from build123d import *

# Parameters (mm, degrees)
SKETCH1_W               = 339.725
SKETCH1_H               = 88.9
BOSS_EXTRUDE1_DEPTH     = 6.35
F_1_4_CLEARANCE_HOLE1_D = 6.7564
FILLET1_R               = 3.175


with BuildPart() as part:
    # Sketch1 → Boss-Extrude1 (new body)
    with BuildSketch(Plane(origin=(0, 0, 0), x_dir=(-1, 0, 0), z_dir=(0, 0, -1))):
        Rectangle(SKETCH1_W, SKETCH1_H)
    extrude(amount=-BOSS_EXTRUDE1_DEPTH)

    # 1/4 Clearance Hole1 (through all)
    with Locations(Plane.XY.offset(6.35)):
        with Locations((-160.3375, 34.925), (-160.3375, -34.925), (160.3375, 34.925), (160.3375, -34.925)):
            Hole(F_1_4_CLEARANCE_HOLE1_D / 2)

    # Fillet1
    fillet1_edges = [part.edges().sort_by_distance(p)[0] for p in [
        (169.8625, 44.45, 3.175),
        (-169.8625, 44.45, 3.175),
        (-169.8625, -44.45, 3.175),
        (169.8625, -44.45, 3.175),
    ]]
    fillet(fillet1_edges, radius=FILLET1_R)


solid = part.part
Could you check a few things on this model? Use its own coordinates, in mm. Coordinates: 2 decimals unless noted, no trailing zeros. Answer in a Markdown table with one row per item. Add a question column.
(1) I need wall thicknesses on L1, parallel to X at y = 32, z = 4.25; L2, parallel to X at y = -37, z = 4.75. Which ranges of each line are inside material? Lowest first, please.
(2) Will this pin go through, and if not, where does the flat tip stop? pin 1 (5.5 mm diameter, centred on x = 160.34, y = 34.92, fed in from -Z).
(3) If we mould it in two halves opening along X, with no side actions, what happens to faces 1 (the face through (2, 1, 0)), 2 (the face through (-169.862, -1, 3)), 3 (the face through (-163.56, -33.91, 3.13))? For each: released by +X, released by -X, zero draft, split by the parting line, or undercut.
Results are:
| question | item | result |
|---|---|---|
| 1 | L1 | x = -169.86 to -162.03, -158.65 to 158.65, 162.03 to 169.86 |
| 1 | L2 | x = -169.86 to -163, -157.67 to 157.67, 163 to 169.86 |
| 2 | pin 1 | passes through |
| 3 | face 1 | zero draft |
| 3 | face 2 | released by -X |
| 3 | face 3 | undercut |
